The listing builds one solid part. Answer for the finished solid, in the listing's coordinates (mm). A direction names the side the tool comes from. Round coordinates to 2 decimals unless told otherwise and drop trailing zeros. Write each loop counter-clockwise with the first axis right and the second up, starting at its lowest first coordinate (ties: lowest second). Pieces come first, ordered by that corner, then holes. Notation, with made-up numbers: M -30.75,12 L 6.25,12 A27 ccw 6.25,32 Z; hole C -36,46 d10. An arc over 180 degrees is marked long. Put each result on its own line as item: value. Start each with the question number.
```python
from build123d import *

# Parameters (mm, degrees)
F1_DEPTH = 12.7


with BuildPart() as f1:
    # F0 (on Front) → F1 (new body)
    with BuildSketch(Plane.XZ):
        with BuildLine():
            Line((0, 76.2), (0, 0))
            Line((0, 0), (71.12, 0))
            ThreePointArc((71.12, 0), (72.5485199348, 3.5317266787), (76.0306666667, 5.0771769934))
            ThreePointArc((76.0306666667, 5.0771769934), (52.0555429955, 55.6476454439), (0, 76.2))
        make_face()
        with BuildLine():
            ThreePointArc((76.0306666667, 5.0771769934), (72.5485199348, 3.5317266787), (71.12, 0))
            Line((71.12, 0), (76.2, 0))
            ThreePointArc((76.2, 0), (76.1576549009, 2.54), (76.0306666667, 5.0771769934))
        make_face()
        with BuildLine():
            ThreePointArc((76.0306666667, 5.0771769934), (76.1576549009, 2.54), (76.2, 0))
            Line((76.2, 0), (81.28, 0))
            ThreePointArc((81.28, 0), (79.7317266787, 3.6514800652), (76.0306666667, 5.0771769934))
        make_face()
        with BuildLine():
            Line((101.6, 76.2), (0, 76.2))
            ThreePointArc((0, 76.2), (52.0555429955, 55.6476454439), (76.0306666667, 5.0771769934))
            ThreePointArc((76.0306666667, 5.0771769934), (79.7317266787, 3.6514800652), (81.28, 0))
            Line((81.28, 0), (101.6, 0))
            Line((101.6, 0), (101.6, 76.2))
        make_face()
    extrude(amount=F1_DEPTH)

    # F3: sweep along a path in F0
    with BuildLine(Plane.XZ) as f3_path:
        ThreePointArc((0, 76.2), (53.8815367264, 53.8815367264), (76.2, 0))
    # F2 (on Top) → F3 (sweep)
    with BuildSketch(Plane.XY):
        with BuildLine():
            ThreePointArc((76.419301331, 0), (71.2296506655, 4.8893362163), (66.04, 0))
            Line((66.04, 0), (76.419301331, 0))
        make_face()
    sweep(path=f3_path.line)


solid = f1.part
```
Item 1: Section A-A (x = 81.5) is taken. Give the vertices of the cut face in (y, z), and give its area (3 significant figures).
Item 2: Which of the six approach directions +Z, -Z, +X, -X, +Y, -Y give full straight-line access (tool end or side, diameter ignored) to faces 1 (the flat face through (101.6, -6, 38)), 2 (the flat face through (74, 0, 47)), 3 (the flat face through (25, 0, 26))?
Item 3: Flat-ended cylindrical pins translate along their axes: pin 1 (1 mm diameter, centred on x = 21.5, z = 60.5, fed in from +Y); pin 2 (2 mm diameter, centred on x = 53.5, y = 2.5, fed in from -Z); pin 3 (6.5 mm diameter, centred on x = 31, y = -7.5, fed in from +Z). Find the tip coordinate at first contact, or state that the pin passes through.
Item 4: Section B-B (y = 3) is taken. Give the vertices of the cut face in (x, z).
Item 5: Consider line 1 along Y through (x, z) = (9, 4); line 2 along Z through (x, y) = (14, -0.75); line 3 along Y through (x, z) = (58.5, 42.5). Determine where each line is inside the solid, lowest interval first. Write a range as [from, to].
Output values:
1. outline: M -12.7,0 L 0,0 L 0,76.2 L -12.7,76.2 Z
1. area: 968 mm^2
2. face 1: +Z, -Z, +X, +Y, -Y
2. face 2: +Z, +X, +Y
2. face 3: -Z, -X, +Y
3. pin 1: stops at y = 0
3. pin 2: stops at z = 38.42
3. pin 3: stops at z = 76.2
4. outline: M 0,67.22 A67.22 cw 67.22,0 L 75.24,0 A75.24 ccw 0,75.24 Z
5. line 1: y = [-12.7, 0]
5. line 2: z = [0, 76.2]
5. line 3: y = [-12.7, 4.78]
